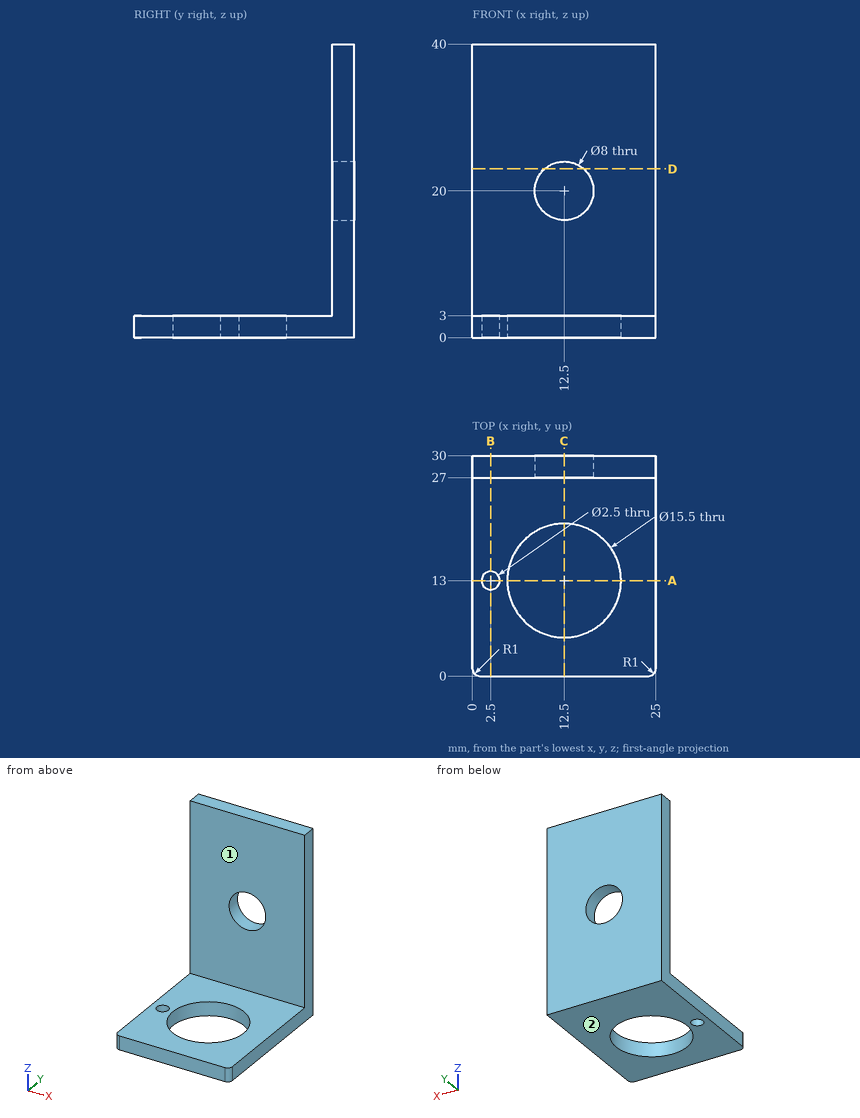
Source: three-view drawing plus pictorial views. Frame: mm from the lowest corner of the part. A direction names the side the tool comes from. Give positions to 0.01 mm unless a question says otherwise; leave off trailing zeros. Write each loop counter-clockwise with the first axis right and the second up, starting at its lowest first coordinate (ties: lowest second). Pieces come first, ordered by that corner, then holes. Notation, with made-up numbers: (40, 30.5) - (96, 30.5) arc R20 cw to (96, 46.5) - close; hole circle Ø10 at (75.5, -20). An arc over 180 degrees is marked (long way). Write item = value, one per line. Start each with the question number.
Q1. Cut plane C-C, the plane x = 12.5. Return loops of the section in (y, z).
Q2. Cut plane D-D, the plane z = 23. Return loops of the section in (x, y).
Q3. Reachability of the marked faces 1 and 2 from +Z, -Z, +X, -X, +Y, -Y: full face, straight path, thin tool, end or side. Return the list, or none.
Q4. Cut plane A-A, the plane y = 13. Return loops of the section in (x, z).
Q5. Cut plane B-B, the plane x = 2.5. Return loops of the section in (y, z), then the cut area to 4 significant figures.
Q6. Pin query (flat end, axial travel): pin 1 Ø12.5 at (x, z) = (7, 20.5) entering from -Y; pin 2 Ø1 at (x, y) = (19, 21) entering from +Z. Return the tip coordinate at first contact, or that it passes through.
Q7. Material intervals for probe 1 along Y at (x, z) = (12.5, 1.7); probe 2 along Y at (x, z) = (7.5, 13); probe 3 along Z at (x, y) = (23.25, 14.5), sorted ascending.
Computed values:
q1.outline = (0, 0) - (5.25, 0) - (5.25, 3) - (0, 3) - close; (20.75, 0) - (30, 0) - (30, 16) - (27, 16) - (27, 3) - (20.75, 3) - close; (27, 24) - (30, 24) - (30, 40) - (27, 40) - close
q2.outline = (0, 27) - (9.85, 27) - (9.85, 30) - (0, 30) - close; (15.15, 27) - (25, 27) - (25, 30) - (15.15, 30) - close
q3.face_1 = +Z, +X, -X, -Y
q3.face_2 = -Z, +X, -X, +Y, -Y
q4.outline = (0, 0) - (1.25, 0) - (1.25, 3) - (0, 3) - close; (3.75, 0) - (4.75, 0) - (4.75, 3) - (3.75, 3) - close; (20.25, 0) - (25, 0) - (25, 3) - (20.25, 3) - close
q5.outline = (0, 0) - (11.75, 0) - (11.75, 3) - (0, 3) - close; (14.25, 0) - (30, 0) - (30, 40) - (27, 40) - (27, 3) - (14.25, 3) - close
q5.area = 193.5 mm²
q6.pin_1 = 27
q6.pin_2 = 3
q7.probe_1 = 0 to 5.25, 20.75 to 30
q7.probe_2 = 27 to 30
q7.probe_3 = 0 to 3
